Design review of the part built by this model. Coordinates are the model's own, in mm. Coordinates: 2 decimals unless noted, no trailing zeros. Loops run counter-clockwise (first coordinate to the right, second up) from the corner with the lowest first, then second, coordinate; pieces in that order, holes last.
Q1. Add section C-C on z = -6. Give the boundary of the cut face in (x, y).
Q2. Add section A-A on y = 3.75. Give the boundary of the cut face in (x, z), and give its area (4 significant figures).
Q3. For P1, Ø0.9, axis at y = -0.5, z = -9, coming from the +X side; P2, Ø1, axis at y = 0, z = -8.5, coming from the -X side; P3, Ø6, axis at x = 6.5, z = -10, coming from the -Y side, all flat-tipped, find the tip position at first contact; note any pin that passes through.
Q4. Wall thickness on probe 1 along X at (y, z) = (3.5, -11); probe 2 along Y at (x, z) = (3, -11); probe 3 along Z at (x, y) = (16, 0.75): over which ranges is each line inside the solid? List them lowest first.
Q5. Add section D-D on y = -0.5. Give the boundary of the cut face in (x, z), and give its area (3 significant figures).
Q6. Add section B-B on x = -2.5. Give the boundary of the cut face in (y, z), and give its area (3 significant figures).
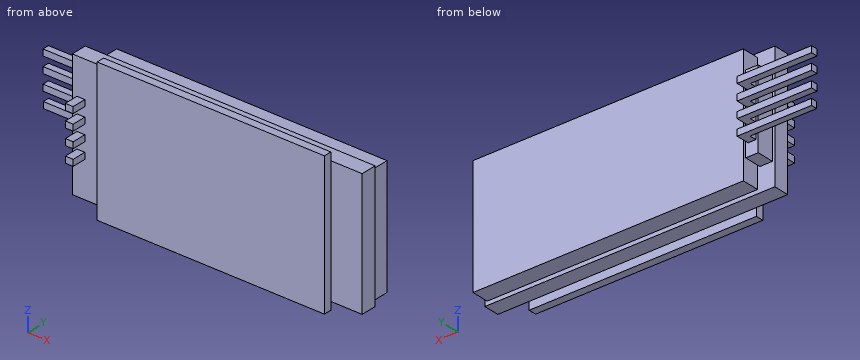
```python
from build123d import *

# Parameters (mm, degrees)
SKETCH1_W                = 37
SKETCH1_H                = 16
BOSS_EXTRUDE1_DEPTH      = 2
SKETCH2_W                = 34.5
SKETCH2_H                = 15
BOSS_EXTRUDE2_DEPTH      = 2.2
SKETCH3_W                = 1.6
SKETCH3_H                = 10
BOSS_EXTRUDE3_DEPTH      = 2.2
SKETCH4_W                = 1
SKETCH4_H                = 0.8
BOSS_EXTRUDE4_DEPTH      = 1.7
BOSS_EXTRUDE4_DEPTH_BACK = 6
SKETCH5_W                = 0.8
SKETCH5_H                = 0.8
SKETCH5_H_2              = 0.85
BOSS_EXTRUDE5_DEPTH      = 8.5
SKETCH6_W                = 29
SKETCH6_H                = 18
BOSS_EXTRUDE6_DEPTH      = 1


with BuildPart() as part:
    # Sketch1 → Boss-Extrude1 (new body)
    with BuildSketch(Plane(origin=(0, 0, 0), x_dir=(1, 0, 0), z_dir=(0, 1, 0))):
        with Locations((18.5, 8)):
            Rectangle(SKETCH1_W, SKETCH1_H)
    extrude(amount=BOSS_EXTRUDE1_DEPTH)

    # Sketch2 → Boss-Extrude2 (add)
    with BuildSketch(Plane(origin=(0, 2, 0), x_dir=(1, 0, 0), z_dir=(0, 1, 0))):
        with Locations((19.45, 8)):
            Rectangle(SKETCH2_W, SKETCH2_H)
    extrude(amount=BOSS_EXTRUDE2_DEPTH)

    # Sketch3 → Boss-Extrude3 (add)
    with BuildSketch(Plane(origin=(0, 2, 0), x_dir=(1, 0, 0), z_dir=(0, 1, 0))):
        with Locations((1.1, 8)):
            Rectangle(SKETCH3_W, SKETCH3_H)
    extrude(amount=BOSS_EXTRUDE3_DEPTH)

    # Sketch4 → Boss-Extrude4 (add, two sides)
    with BuildSketch(Plane(origin=(0, 4.2, 0), x_dir=(1, 0, 0), z_dir=(0, 1, 0))) as boss_extrude4_sk:
        with Locations((1.1, 11)):
            Rectangle(SKETCH4_W, SKETCH4_H)
        with Locations((1.1, 9)):
            Rectangle(SKETCH4_W, SKETCH4_H)
        with Locations((1.1, 7)):
            Rectangle(SKETCH4_W, SKETCH4_H)
        with Locations((1.1, 5)):
            Rectangle(SKETCH4_W, SKETCH4_H)
    extrude(amount=BOSS_EXTRUDE4_DEPTH)
    extrude(boss_extrude4_sk.sketch, amount=-BOSS_EXTRUDE4_DEPTH_BACK)

    # Sketch5 → Boss-Extrude5 (add)
    with BuildSketch(Plane.ZY.offset(-0.6)):
        with Locations((-11, 5.5)):
            Rectangle(SKETCH5_W, SKETCH5_H)
        with Locations((-9, 5.475)):
            Rectangle(SKETCH5_W, SKETCH5_H_2)
        with Locations((-7, 5.475)):
            Rectangle(SKETCH5_W, SKETCH5_H_2)
        with Locations((-5, 5.475)):
            Rectangle(SKETCH5_W, SKETCH5_H_2)
    extrude(amount=BOSS_EXTRUDE5_DEPTH)

    # Sketch6 → Boss-Extrude6 (add)
    with BuildSketch(Plane(origin=(0, 0, 0), x_dir=(-1, 0, 0), z_dir=(0, -1, 0))):
        with Locations((-18.5, 8)):
            Rectangle(SKETCH6_W, SKETCH6_H)
    extrude(amount=BOSS_EXTRUDE6_DEPTH)


solid = part.part
```
Entries:
1. outline: (0, 0) - (4, 0) - (4, -1) - (33, -1) - (33, 0) - (37, 0) - (37, 2) - (36.7, 2) - (36.7, 4.2) - (2.2, 4.2) - (2.2, 2) - (1.9, 2) - (1.9, 4.2) - (0.3, 4.2) - (0.3, 2) - (0, 2) - close
2. outline: (0.3, -13) - (1.9, -13) - (1.9, -3) - (0.3, -3) - close; (2.2, -15.5) - (36.7, -15.5) - (36.7, -0.5) - (2.2, -0.5) - close
2. area: 533.5 mm2
3. P1: stops at x = 33
3. P2: stops at x = 0
3. P3: stops at y = -1
4. probe 1: x = 0.3 to 1.9, 2.2 to 36.7
4. probe 2: y = 0 to 4.2
4. probe 3: z = -16 to 0
5. outline: (0.6, -11.4) - (1.6, -11.4) - (1.6, -10.6) - (0.6, -10.6) - close; (0.6, -9.4) - (1.6, -9.4) - (1.6, -8.6) - (0.6, -8.6) - close; (0.6, -7.4) - (1.6, -7.4) - (1.6, -6.6) - (0.6, -6.6) - close; (0.6, -5.4) - (1.6, -5.4) - (1.6, -4.6) - (0.6, -4.6) - close; (4, -17) - (33, -17) - (33, 1) - (4, 1) - close
5. area: 525 mm2
6. outline: (5.05, -9.4) - (5.9, -9.4) - (5.9, -8.6) - (5.05, -8.6) - close; (5.05, -7.4) - (5.9, -7.4) - (5.9, -6.6) - (5.05, -6.6) - close; (5.05, -5.4) - (5.9, -5.4) - (5.9, -4.6) - (5.05, -4.6) - close; (5.1, -11.4) - (5.9, -11.4) - (5.9, -10.6) - (5.1, -10.6) - close
6. area: 2.68 mm2
